from build123d import *

# Parameters (mm, degrees)
F2_DEPTH = 1.7
F3_DEPTH = 2
F5_DEPTH = 0.9


with BuildPart() as f2:
    # F0 (on Top) → F2 (new body)
    with BuildSketch(Plane.XY):
        with BuildLine():
            Line((1.5, 7.5), (-9, 7.5))
            Line((-9, 7.5), (-9, 6.3))
            Line((-9, 6.3), (-7.9, 5.8))
            Line((-7.9, 5.8), (-7.4, 5.8))
            Line((-7.4, 5.8), (-7.4, 6.3))
            Line((-7.4, 6.3), (-4.7, 6.3))
            Line((-4.7, 6.3), (-4.7, 4.5))
            Line((-4.7, 4.5), (-4.7, -6.3))
            Line((-4.7, -6.3), (-7.4, -6.3))
            Line((-7.4, -6.3), (-7.4, -5.8))
            Line((-7.4, -5.8), (-7.9, -5.8))
            Line((-7.9, -5.8), (-9, -6.3))
            Line((-9, -6.3), (-9, -7.5))
            Line((-9, -7.5), (1.5, -7.5))
            ThreePointArc((1.5, -7.5), (9, 0), (1.5, 7.5))
        make_face()
    extrude(amount=F2_DEPTH)

    # F1 (on Top) → F3 (cut)
    with BuildSketch(Plane.XY):
        with BuildLine():
            Line((-4.7, -5.5), (-4.7, -4.582576))
            ThreePointArc((-4.7, -4.582576), (-1.7, 0), (-4.7, 4.582576))
            Line((-4.7, 4.582576), (-4.7, 5.5))
            Line((-4.7, 5.5), (-13.7, 5.5))
            Line((-13.7, 5.5), (-13.7, -5.5))
            Line((-13.7, -5.5), (-4.7, -5.5))
        make_face()
    extrude(amount=F3_DEPTH, mode=Mode.SUBTRACT)

    # F4 (on face) → F5 (join)
    with BuildSketch(Plane.XY.offset(1.7)):
        with BuildLine():
            Line((-0.35, 7.5), (-8.25, 7.5))
            ThreePointArc((-8.25, 7.5), (-8.7, 7.05), (-8.25, 6.6))
            Line((-8.25, 6.6), (-0.35, 6.6))
            ThreePointArc((-0.35, 6.6), (0.1, 7.05), (-0.35, 7.5))
        make_face()
        with BuildLine():
            Line((-0.35, -6.6), (-8.25, -6.6))
            ThreePointArc((-8.25, -6.6), (-8.7, -7.05), (-8.25, -7.5))
            Line((-8.25, -7.5), (-0.35, -7.5))
            ThreePointArc((-0.35, -7.5), (0.1, -7.05), (-0.35, -6.6))
        make_face()
    extrude(amount=F5_DEPTH)


solid = f2.part
Read the model definition and answer for the solid it produces. Units are mm, in the model's axes. A direction names the side the tool comes from. Give positions to 0.01 mm unless a question says otherwise; leave off trailing zeros. Write each loop counter-clockwise with the first axis right and the second up, starting at its lowest first coordinate (ties: lowest second). Pieces come first, ordered by that corner, then holes. Notation, with made-up numbers: (32.25, -12) -> (51.25, -12) arc R8 ccw to (51.25, -4) -> close; hole circle Ø1 at (-26, -23). An arc over 180 degrees is marked (long way). Answer as a JSON object with one key per item and string values. Group by question number.
1) Find section D-D (x = -3.5). Write down the section's boundary in (y, z).
2) Find section C-C (y = 7.05). Write down the section's boundary in (x, z), and give its area (3 significant figures).
3) Find section A-A (x = -6.5). Write down the section's boundary in (y, z).
4) Consider L1, parallel to Y at x = -6.5, z = 1.45; L2, parallel to Z at x = 3.5, y = -6; L3, parallel to Y at x = -6.75, z = 2. Determine where each line is inside the solid, lowest interval first. Write a range as from..to.
5) Each of these flat-tipped pins is pushed along its axis until it touches: P1, Ø2, axis at x = -5, y = 2, coming from the +Z side; P2, Ø0.8, axis at y = -5, z = 1, coming from the -X side; P3, Ø0.6, axis at y = 6, z = 1, coming from the +X side. Where does it stop, or does it pass through?
6) Find section B-B (z = 2.1). Write down the section's boundary in (x, y).
7) A tool of negligible diameter and unlimited length cuts with its end or side. For faces 5 (the flat face through (-4.7, -5, 1)), 6 (the cylindrical face through (0.1, 7.04, 2.14)), 7 (the cylindrical face through (-8.7, 7.06, 2.14)), 8 (the flat face through (-8.458, 6.054, 0.838)), 9 (the flat face through (-4, -6.6, 2)), from which of +Z, -Z, +X, -X, +Y, -Y can it reach the whole face along a straight path? Write none if from no direction.
8) The mould has two halves that part along Y. Classify faces 1 (the flat face through (-4, -7, 2.6)), 2 (the flat face through (-4, -7.5, 1)), 3 (the flat face through (-4, 7.5, 1)), 4 (the flat face through (-4.7, 5, 1)): +Y half, -Y half, draft (parallel to the pull), parting line (faces both ways), or undercut.
Values follow:
{
 "1": {"outline": "(-7.5, 0) -> (-3.84, 0) -> (-3.84, 1.7) -> (-6.6, 1.7) -> (-6.6, 2.6) -> (-7.5, 2.6) -> close; (3.84, 0) -> (7.5, 0) -> (7.5, 2.6) -> (6.6, 2.6) -> (6.6, 1.7) -> (3.84, 1.7) -> close"},
 "2": {"outline": "(-9, 0) -> (4.06, 0) -> (4.06, 1.7) -> (0.1, 1.7) -> (0.1, 2.6) -> (-8.7, 2.6) -> (-8.7, 1.7) -> (-9, 1.7) -> close", "area": "30.1 mm2"},
 "3": {"outline": "(-7.5, 0) -> (-6.3, 0) -> (-6.3, 1.7) -> (-6.6, 1.7) -> (-6.6, 2.6) -> (-7.5, 2.6) -> close; (6.3, 0) -> (7.5, 0) -> (7.5, 2.6) -> (6.6, 2.6) -> (6.6, 1.7) -> (6.3, 1.7) -> close"},
 "4": {"L1": "y = -7.5..-6.3, 6.3..7.5", "L2": "z = 0..1.7", "L3": "y = -7.5..-6.6, 6.6..7.5"},
 "5": {"P1": "passes through", "P2": "stops at x = -4.7", "P3": "stops at x = 6.37"},
 "6": {"outline": "(-8.25, -7.5) -> (-0.35, -7.5) arc R0.45 ccw to (-0.35, -6.6) -> (-8.25, -6.6) arc R0.45 ccw to start; (-8.25, 6.6) -> (-0.35, 6.6) arc R0.45 ccw to (-0.35, 7.5) -> (-8.25, 7.5) arc R0.45 ccw to start"},
 "7": {"face 5": "+Z, -Z", "face 6": "+Z, +X", "face 7": "+Z, -X", "face 8": "+Z, -Z, -X", "face 9": "+Z, +X, -X"},
 "8": {"face 1": "draft", "face 2": "-Y half", "face 3": "+Y half", "face 4": "undercut"}
}
